```python
from build123d import *

# Parameters (mm, degrees)
BOX001_W        = 5
BOX001_H        = 5
BOX001_DEPTH    = 1
BOX002_W        = 6.8
BOX002_H        = 6.8
BOX002_DEPTH    = 0.5
BOX_W           = 7
BOX_H           = 7
BOX_DEPTH       = 5.5
SKETCH_W        = 1
SKETCH_H        = 6
POCKET_DEPTH    = 0.5
SKETCH001_W     = 1
SKETCH001_H     = 6
POCKET001_DEPTH = 0.5
SKETCH002_W     = 0.4
SKETCH002_H     = 0.5
PAD_DEPTH       = 6


with BuildPart() as obj1:
    # Sphere001 → Sphere001 (revolve)
    with BuildSketch(Plane(origin=(4.9, 3.5, 5), x_dir=(1, 0, 0), z_dir=(0, -1, 0))):
        with BuildLine():
            ThreePointArc((0, -0.9), (0.9, 0), (0, 0.9))
            Line((0, 0.9), (0, -0.9))
        make_face()
    revolve(axis=Axis((4.9, 3.5, 5), (0, 0, 1)))


with BuildPart() as obj2:
    # Sphere → Sphere (revolve)
    with BuildSketch(Plane(origin=(2.1, 3.5, 5), x_dir=(1, 0, 0), z_dir=(0, -1, 0))):
        with BuildLine():
            ThreePointArc((0, -0.9), (0.9, 0), (0, 0.9))
            Line((0, 0.9), (0, -0.9))
        make_face()
    revolve(axis=Axis((2.1, 3.5, 5), (0, 0, 1)))


with BuildPart() as cubo001:
    # Box001 → Box001 (new body)
    with BuildSketch(Plane(origin=(1, 1, 5), x_dir=(1, 0, 0), z_dir=(0, 0, 1))):
        with Locations((2.5, 2.5)):
            Rectangle(BOX001_W, BOX001_H)
    extrude(amount=BOX001_DEPTH)


with BuildPart() as cubo002:
    # Box002 → Box002 (new body)
    with BuildSketch(Plane(origin=(0.1, 0.1, 5.5), x_dir=(1, 0, 0), z_dir=(0, 0, 1))):
        with Locations((3.4, 3.4)):
            Rectangle(BOX002_W, BOX002_H)
    extrude(amount=BOX002_DEPTH)


with BuildPart() as obj3:
    # Box → Box (new body)
    with BuildSketch(Plane.XY):
        with Locations((3.5, 3.5)):
            Rectangle(BOX_W, BOX_H)
    extrude(amount=BOX_DEPTH)

    # Fusion: union Cubo002
    add(cubo002.part)

    # Cut: cut Cubo001
    add(cubo001.part, mode=Mode.SUBTRACT)

    # Sketch → Pocket (cut)
    with BuildSketch(Plane.XZ):
        with Locations((3.5, 3)):
            Rectangle(SKETCH_W, SKETCH_H)
    extrude(amount=-POCKET_DEPTH, mode=Mode.SUBTRACT)

    # Sketch001 → Pocket001 (cut)
    with BuildSketch(Plane(origin=(0, 7, 0), x_dir=(-1, 0, 0), z_dir=(0, 1, 0))):
        with Locations((-3.5, 3)):
            Rectangle(SKETCH001_W, SKETCH001_H)
    extrude(amount=-POCKET001_DEPTH, mode=Mode.SUBTRACT)

    # Sketch002 → Pad (new body)
    with BuildSketch(Plane(origin=(0, 0, 0), x_dir=(1, 0, 0), z_dir=(0, 0, -1))):
        with Locations((2.2, -2.1)):
            Rectangle(SKETCH002_W, SKETCH002_H)
        with Locations((4.9, -2.1)):
            Rectangle(SKETCH002_W, SKETCH002_H)
        with Locations((4.9, -4.9)):
            Rectangle(SKETCH002_W, SKETCH002_H)
        with Locations((2.2, -4.9)):
            Rectangle(SKETCH002_W, SKETCH002_H)
    extrude(amount=PAD_DEPTH)

    # Fusion001: union obj1, obj2
    add(obj1.part)
    add(obj2.part)


solid = obj3.part
```
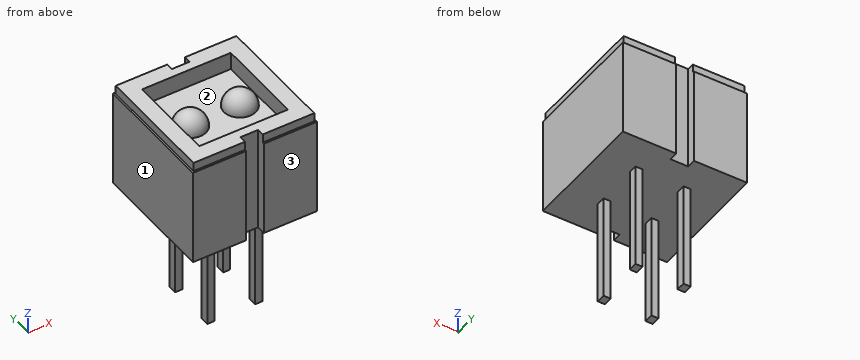
For this review, take the finished solid that the model builds, in its own axes (mm). Face numbers are marked on the shaded views. Give positions to 0.01 mm unless a question says otherwise; leave off trailing zeros. Order: outer loops, then holes, each group sorted by start corner. A loop starts at its lowest first (then second) coordinate and runs counter-clockwise, first axis right, second up.
1) The part is to be moulded in two halves that separate along Y. For the marked faces 1, 2 and 3, say which applies: released by +Y, released by -Y, zero draft, split by the parting line, or undercut.
2) Take a section at C-C (y = 6.25). Give the boundary of the cut face in (x, z).
3) Take a section at A-A (x = 3.75). Give the boundary of the cut face in (y, z), then the cut area to 3 significant figures.
4) Wall thickness on line 1 (Y direction, x = 2.25, z = -1.25); line 2 (Z direction, x = 5.25, y = 4.5); line 3 (Z direction, x = 0.75, y = 6.75): over which ranges is each line inside the solid? List them lowest first.
5) Insertion check: pin 1 (3 mm diameter, centred on x = 1.5, z = -2.5, fed in from +Y); pin 2 (0.6 mm diameter, centred on y = 5, z = -3, fed in from -X); pin 3 (0.8 mm diameter, centred on x = 3.5, z = 1.5, fed in from -Y); pin 4 (1.5 mm diameter, centred on y = 1.5, z = 4.5, fed in from -X). Each pin has a flat end and moves straight along its axis. Give the tip position at first contact, or say it passes through.
6) Take a section at B-B (z = 3). Give the boundary of the cut face in (x, y).
7) Take a section at D-D (y = 1.25). Give the boundary of the cut face in (x, z).
Derived:
1. face 1: zero draft
1. face 2: undercut
1. face 3: released by -Y
2. outline: (0, 0) - (7, 0) - (7, 5.5) - (6.9, 5.5) - (6.9, 6) - (0.1, 6) - (0.1, 5.5) - (0, 5.5) - close
3. outline: (0.5, 0) - (6.5, 0) - (6.5, 6) - (6, 6) - (6, 5) - (1, 5) - (1, 6) - (0.5, 6) - close
3. area: 31.0 mm2
4. line 1: y = 1.85 to 2.35, 4.65 to 5.15
4. line 2: z = 0 to 5
4. line 3: z = 0 to 6
5. pin 1: stops at y = 5.15
5. pin 2: stops at x = 2
5. pin 3: stops at y = 0.5
5. pin 4: stops at x = 0
6. outline: (0, 0) - (3, 0) - (3, 0.5) - (4, 0.5) - (4, 0) - (7, 0) - (7, 7) - (4, 7) - (4, 6.5) - (3, 6.5) - (3, 7) - (0, 7) - close
7. outline: (0, 0) - (7, 0) - (7, 5.5) - (6.9, 5.5) - (6.9, 6) - (6, 6) - (6, 5) - (1, 5) - (1, 6) - (0.1, 6) - (0.1, 5.5) - (0, 5.5) - close
